from build123d import *

# Parameters (mm, degrees)
SKETCH1_W             = 8
SKETCH1_H             = 36
SKETCH1_R             = 1.25
BOSS_EXTRUDE1_DEPTH   = 5
BOSS_EXTRUDE1_2_DEPTH = 5
SKETCH2_W             = 54
SKETCH2_H             = 5
BOSS_EXTRUDE2_DEPTH   = 12
SKETCH4_W             = 54
SKETCH4_H             = 12
BOSS_EXTRUDE3_DEPTH   = 64
SKETCH5_W             = 40.6
SKETCH5_H             = 60.5
CUT_EXTRUDE1_DEPTH    = 10
BOSS_EXTRUDE4_DEPTH   = 3
BOSS_EXTRUDE5_START   = -54
BOSS_EXTRUDE5_DEPTH   = 3
CHAMFER1_SIZE         = 2
CHAMFER2_SIZE         = 1
CHAMFER3_SIZE         = 3
SKETCH8_W             = 66
SKETCH8_H             = 71
BOSS_EXTRUDE6_DEPTH   = 3
SKETCH9_W             = 3
SKETCH9_H             = 46
SKETCH9_W_2           = 4
SKETCH9_H_2           = 71
BOSS_EXTRUDE7_DEPTH   = 6
BOSS_EXTRUDE8_DEPTH   = 40
SKETCH12_W            = 2.5
SKETCH12_H            = 71
BOSS_EXTRUDE9_DEPTH   = 3
CHAMFER4_SIZE         = 5


with BuildPart() as part:
    # Sketch1 → Boss-Extrude1 (new body)
    with BuildSketch(Plane.XY):
        with Locations((1, 15)):
            Rectangle(SKETCH1_W, SKETCH1_H)
        Circle(SKETCH1_R, mode=Mode.SUBTRACT)
        with Locations((0, 30)):
            Circle(SKETCH1_R, mode=Mode.SUBTRACT)
    extrude(amount=BOSS_EXTRUDE1_DEPTH)



with BuildPart() as body_2:
    # Sketch1 → Boss-Extrude1 2 (new body)
    with BuildSketch(Plane.XY):
        with Locations((47, 15)):
            Rectangle(SKETCH1_W, SKETCH1_H)
        with Locations((48, 0)):
            Circle(SKETCH1_R, mode=Mode.SUBTRACT)
        with Locations((48, 30)):
            Circle(SKETCH1_R, mode=Mode.SUBTRACT)
    extrude(amount=BOSS_EXTRUDE1_2_DEPTH)


with BuildPart() as part_1:
    add(part.part)

    add(body_2.part)  # Boss-Extrude2 merges body 2
    # Sketch2 → Boss-Extrude2 (add)
    with BuildSketch(Plane.XZ.offset(3)):
        with Locations((24, 2.5)):
            Rectangle(SKETCH2_W, SKETCH2_H)
    extrude(amount=BOSS_EXTRUDE2_DEPTH)

    # Sketch4 → Boss-Extrude3 (add)
    with BuildSketch(Plane.XY.offset(5)):
        with Locations((24, -9)):
            Rectangle(SKETCH4_W, SKETCH4_H)
    extrude(amount=BOSS_EXTRUDE3_DEPTH)

    # Sketch5 → Cut-Extrude1 (cut)
    with BuildSketch(Plane(origin=(0, -3, 0), x_dir=(1, 0, 0), z_dir=(0, 1, 0))):
        with Locations((24, -39.25)):
            Rectangle(SKETCH5_W, SKETCH5_H)
    extrude(amount=-CUT_EXTRUDE1_DEPTH, mode=Mode.SUBTRACT)

    # Sketch7 → Boss-Extrude4 (add)
    with BuildSketch(Plane.ZY.offset(3)):
        Polygon((0, 33), (0, -15), (48, -15), (48, -3), (5, 33), align=None)
    extrude(amount=BOSS_EXTRUDE4_DEPTH)

    # Sketch7<2> → Boss-Extrude5 (add)
    with BuildSketch(Plane.ZY.offset(3).offset(BOSS_EXTRUDE5_START)):
        Polygon((0, 33), (0, -15), (48, -15), (48, -3), (5, 33), align=None)
    extrude(amount=-BOSS_EXTRUDE5_DEPTH)

    # Chamfer1
    chamfer1_edges = [part_1.edges().sort_by_distance(p)[0] for p in [
        (-3, -9, 69),
        (51, -9, 69),
        (-6, 9, 0),
        (54, 9, 0),
    ]]
    chamfer(chamfer1_edges, length=CHAMFER1_SIZE)

    # Chamfer2
    chamfer2_edges = [part_1.edges().sort_by_distance(p)[0] for p in [
        (44.3, -3, 39),
        (24, -3, 9),
        (3.7, -3, 39),
    ]]
    chamfer(chamfer2_edges, length=CHAMFER2_SIZE)

    # Chamfer3
    # the kernel refuses this chamfer: 3 mm, written as the material it adds along each edge
    with BuildSketch(Plane(origin=(51, -15, 48), x_dir=(-0.027495876610584467, 0, 0.9996219169112969), z_dir=(0, 1, 0))) as chamfer3_piece_1_section:
        Polygon((CHAMFER3_SIZE * 0.999621916911, CHAMFER3_SIZE * 0.0274958766106), (-CHAMFER3_SIZE * 0.0274958766106, CHAMFER3_SIZE * 0.999621916911), (0, 0), align=None)
    chamfer3_piece_1 = extrude(amount=12, mode=Mode.PRIVATE)
    chamfer3_piece_1 = split(chamfer3_piece_1, bisect_by=Plane(origin=(54, -9.397887016, 48.948587344), z_dir=(-1, 0, 0)), keep=Keep.TOP, mode=Mode.PRIVATE)
    chamfer3_piece_1 = split(chamfer3_piece_1, bisect_by=Plane(origin=(52.008422093, -6.10336241, 51.70679399), z_dir=(0, -0.7667576729931039, -0.6419366564593428)), keep=Keep.TOP, mode=Mode.PRIVATE)
    add(chamfer3_piece_1)
    with BuildSketch(Plane(origin=(51, -15, 48), x_dir=(-0.027495876610584467, 0, 0.9996219169112969), z_dir=(0, 1, 0))) as chamfer3_piece_2_section:
        Polygon((CHAMFER3_SIZE * 0.999621916911, CHAMFER3_SIZE * 0.0274958766106), (-CHAMFER3_SIZE * 0.0274958766106, CHAMFER3_SIZE * 0.999621916911), (0, 0), align=None)
    chamfer3_piece_2 = extrude(amount=12, mode=Mode.PRIVATE)
    chamfer3_piece_2 = split(chamfer3_piece_2, bisect_by=Plane(origin=(51.683373084, -4.039508932, 49.241635668), z_dir=(0, 0.7667576729931039, 0.6419366564593428)), keep=Keep.TOP, mode=Mode.PRIVATE)
    add(chamfer3_piece_2)
    with BuildSketch(Plane(origin=(-3, -15, 48), x_dir=(0.027495876610586334, 0, 0.9996219169112968), z_dir=(0, 1, 0))) as chamfer3_piece_3_section:
        Polygon((CHAMFER3_SIZE * 0.999621916911, -CHAMFER3_SIZE * 0.0274958766106), (-CHAMFER3_SIZE * 0.0274958766106, -CHAMFER3_SIZE * 0.999621916911), (0, 0), align=None)
    chamfer3_piece_3 = extrude(amount=12, mode=Mode.PRIVATE)
    chamfer3_piece_3 = split(chamfer3_piece_3, bisect_by=Plane(origin=(-6, -9.397887016, 48.948587344), z_dir=(1, 0, 0)), keep=Keep.TOP, mode=Mode.PRIVATE)
    chamfer3_piece_3 = split(chamfer3_piece_3, bisect_by=Plane(origin=(-4.008422093, -6.10336241, 51.70679399), z_dir=(0, -0.7667576729931039, -0.6419366564593428)), keep=Keep.TOP, mode=Mode.PRIVATE)
    add(chamfer3_piece_3)
    with BuildSketch(Plane(origin=(-3, -15, 48), x_dir=(0.027495876610586334, 0, 0.9996219169112968), z_dir=(0, 1, 0))) as chamfer3_piece_4_section:
        Polygon((CHAMFER3_SIZE * 0.999621916911, -CHAMFER3_SIZE * 0.0274958766106), (-CHAMFER3_SIZE * 0.0274958766106, -CHAMFER3_SIZE * 0.999621916911), (0, 0), align=None)
    chamfer3_piece_4 = extrude(amount=12, mode=Mode.PRIVATE)
    chamfer3_piece_4 = split(chamfer3_piece_4, bisect_by=Plane(origin=(-3.683373084, -4.039508932, 49.241635668), z_dir=(0, 0.7667576729931039, 0.6419366564593428)), keep=Keep.TOP, mode=Mode.PRIVATE)
    add(chamfer3_piece_4)
    with BuildSketch(Plane(origin=(-3, 33, 5), x_dir=(-0.02749587661058635, 0, 0.9996219169112968), z_dir=(0, -1, 0))) as chamfer3_piece_5_section:
        Polygon((CHAMFER3_SIZE * 0.999621916911, -CHAMFER3_SIZE * 0.0274958766106), (-CHAMFER3_SIZE * 0.0274958766106, -CHAMFER3_SIZE * 0.999621916911), (0, 0), align=None)
    chamfer3_piece_5 = extrude(amount=43.715048964, mode=Mode.PRIVATE)
    chamfer3_piece_5 = split(chamfer3_piece_5, bisect_by=Plane(origin=(-2.02772284, 24.92424675, 14.646038604), z_dir=(0, -0.7667576729931039, -0.6419366564593428)), keep=Keep.TOP, mode=Mode.PRIVATE)
    chamfer3_piece_5 = chamfer3_piece_5 - Plane(origin=(0, 0, 5.988374144), x_dir=(1, 0, 0), z_dir=(0, 0, -1)) * Cylinder(1.25, 100, mode=Mode.PRIVATE)
    chamfer3_piece_5 = chamfer3_piece_5 - Plane(origin=(0, 30, 5.988374144), x_dir=(1, 0, 0), z_dir=(0, 0, -1)) * Cylinder(1.25, 100, mode=Mode.PRIVATE)
    add(chamfer3_piece_5)
    with BuildSketch(Plane(origin=(51, -10.715048964, 5), x_dir=(0.02749587661058678, 0, 0.9996219169112968), z_dir=(0, 1, 0))) as chamfer3_piece_6_section:
        Polygon((CHAMFER3_SIZE * 0.999621916911, -CHAMFER3_SIZE * 0.0274958766106), (-CHAMFER3_SIZE * 0.0274958766106, -CHAMFER3_SIZE * 0.999621916911), (0, 0), align=None)
    chamfer3_piece_6 = extrude(amount=43.715048964, mode=Mode.PRIVATE)
    chamfer3_piece_6 = split(chamfer3_piece_6, bisect_by=Plane(origin=(50.01061912, 16.088421834, 25.199940587), z_dir=(0, -0.7667576729931039, -0.6419366564593428)), keep=Keep.TOP, mode=Mode.PRIVATE)
    chamfer3_piece_6 = chamfer3_piece_6 - Plane(origin=(48, 0, 5.98938088), x_dir=(1, 0, 0), z_dir=(0, 0, -1)) * Cylinder(1.25, 100, mode=Mode.PRIVATE)
    chamfer3_piece_6 = chamfer3_piece_6 - Plane(origin=(48, 30, 5.98938088), x_dir=(1, 0, 0), z_dir=(0, 0, -1)) * Cylinder(1.25, 100, mode=Mode.PRIVATE)
    add(chamfer3_piece_6)

    # Sketch8 → Boss-Extrude6 (add)
    with BuildSketch(Plane.XZ.offset(15)):
        with Locations((82, 35.5)):
            Rectangle(SKETCH8_W, SKETCH8_H)
    extrude(amount=-BOSS_EXTRUDE6_DEPTH)

    # Sketch9 → Boss-Extrude7 (add)
    with BuildSketch(Plane(origin=(0, -12, 0), x_dir=(1, 0, 0), z_dir=(0, 1, 0))):
        with Locations((55.5, -25)):
            Rectangle(SKETCH9_W, SKETCH9_H)
        with Locations((113, -35.5)):
            Rectangle(SKETCH9_W_2, SKETCH9_H_2)
    extrude(amount=BOSS_EXTRUDE7_DEPTH)

    # Sketch11 → Boss-Extrude8 (add)
    with BuildSketch(Plane(origin=(0, 0, 2), x_dir=(-1, 0, 0), z_dir=(0, 0, -1))):
        with BuildLine():
            Line((-54, -1.45), (-54, -4.65))
            ThreePointArc((-54, -4.65), (-54.8, -3.05), (-54, -1.45))
        make_face()
    extrude(amount=-BOSS_EXTRUDE8_DEPTH)

    # Sketch12 → Boss-Extrude9 (add)
    with BuildSketch(Plane(origin=(0, -6, 0), x_dir=(1, 0, 0), z_dir=(0, 1, 0))):
        with Locations((113.75, -35.5)):
            Rectangle(SKETCH12_W, SKETCH12_H)
    extrude(amount=BOSS_EXTRUDE9_DEPTH)

    # Chamfer4
    # the kernel refuses this chamfer: 5 mm, written as the material it takes off along each edge
    with BuildSketch(Plane(origin=(115, -12, 0), x_dir=(-0.9996219169112968, 0, -0.027495876610586334), z_dir=(0, 1, 0))) as chamfer4_piece_1:
        Polygon((CHAMFER4_SIZE * 0.999621916911, CHAMFER4_SIZE * 0.0274958766106), (-CHAMFER4_SIZE * 0.0274958766106, CHAMFER4_SIZE * 0.999621916911), (0, 0), align=None)
    extrude(amount=6, mode=Mode.SUBTRACT)
    with BuildSketch(Plane(origin=(115, -12, 71), x_dir=(-0.9996219169112968, 0, 0.027495876610587663), z_dir=(0, 1, 0))) as chamfer4_piece_2:
        Polygon((CHAMFER4_SIZE * 0.999621916911, -CHAMFER4_SIZE * 0.0274958766106), (-CHAMFER4_SIZE * 0.0274958766106, -CHAMFER4_SIZE * 0.999621916911), (0, 0), align=None)
    extrude(amount=6, mode=Mode.SUBTRACT)
    with BuildSketch(Plane(origin=(115, -27.85841494, 71), x_dir=(-0.9996219169112968, 0, 0.027495876610587663), z_dir=(0, 1, 0)), Plane(origin=(115, -6, 71), x_dir=(-0.9996219169112968, 0, 0.027495876610587663), z_dir=(0, 1, 0))) as chamfer4_piece_3:
        Polygon((CHAMFER4_SIZE * 0.999621916911, -CHAMFER4_SIZE * 0.0274958766106), (-CHAMFER4_SIZE * 0.0274958766106, -CHAMFER4_SIZE * 0.999621916911), (0, 0), align=None)
    extrude(amount=15.85841494, mode=Mode.SUBTRACT)
    with BuildSketch(Plane(origin=(115, -27.85841494, 0), x_dir=(-0.9996219169112968, 0, -0.02749587661058646), z_dir=(0, 1, 0)), Plane(origin=(115, -6, 0), x_dir=(-0.9996219169112968, 0, -0.02749587661058634), z_dir=(0, 1, 0))) as chamfer4_piece_4:
        Polygon((CHAMFER4_SIZE * 0.999621916911, CHAMFER4_SIZE * 0.0274958766106), (-CHAMFER4_SIZE * 0.0274958766106, CHAMFER4_SIZE * 0.999621916911), (0, 0), align=None)
    extrude(amount=15.85841494, mode=Mode.SUBTRACT)


solid = part_1.part
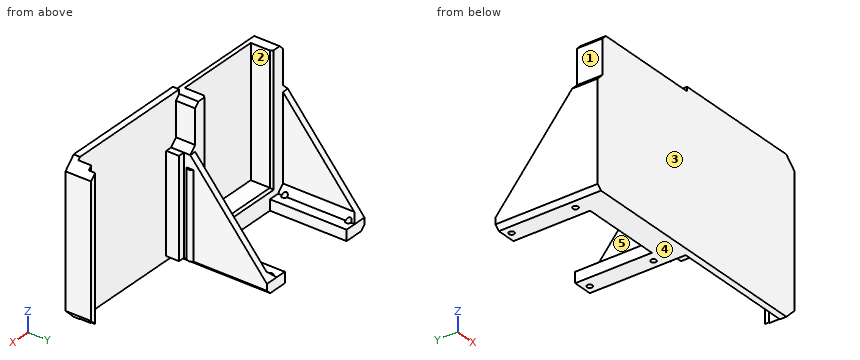
Geometry: final body of the model. Coordinates: model frame, mm. Face numbers are marked on the shaded views. A direction names the side the tool comes from. Round coordinates to 2 decimals unless told otherwise and drop trailing zeros. Order: outer loops, then holes, each group sorted by start corner. A loop starts at its lowest first (then second) coordinate and runs counter-clockwise, first axis right, second up. Notation, with made-up numbers: (-32, 54) -> (5, 54) arc R13 cw to (5, 59) -> close; hole circle Ø8 at (16.5, 60.5). An arc over 180 degrees is marked (long way). Put each result on its own line as item: value. Start each with the question number.
Q1. First-contact query: pin 1 (4 mm diameter, centred on x = 3.5, y = 17, fed in from +Z); pin 2 (1.5 mm diameter, centred on x = 0, y = 30, fed in from -Z); pin 3 (3.5 mm diameter, centred on x = 16, y = -12, fed in from +Z); pin 4 (1 mm diameter, centred on y = -13.5, z = 70, fed in from -X). Flat tips, straight axial feed; report the tip coordinate or a pass-through.
Q2. Line query: probe 1 along X at (y, z) = (30, 3.45); probe 2 along X at (y, z) = (-11, 38); probe 3 along Y at (x, z) = (48, 1.75). Output: solid intervals per line, ascending.
Q3. Section A-A on y = 15. Return the cut outline in (x, z), and give its area (3 significant figures).
Q4. Section C-C on z = 23. Return the cut outline in (x, y).
Q5. Reachability of the marked faces 4 and 5 from +Z, -Z, +X, -X, +Y, -Y: full face, straight path, thin tool, end or side. Return the list, or none.
Q6. Section D-D on y = 7.5. Return the cut outline in (x, z), and give its area (3 significant figures).
Q7. Section B-B on y = 0. Return the cut outline in (x, z), and give its area (3 significant figures).
Q8. Pull-direction query (X, two-part tool) for the marked faces 1, 2 and 3; classes: +X half, -X half, draft (parallel to the pull), parting line (faces both ways), or undercut.
Ans:
1. pin 1: stops at z = 5
1. pin 2: passes through
1. pin 3: stops at z = 69
1. pin 4: stops at x = 49
2. probe 1: x = -6 to -1.25, 1.25 to 5, 43 to 46.75, 49.25 to 54
2. probe 2: x = -6 to 3.7, 44.3 to 57, 111 to 115
2. probe 3: y = -15 to -1.25, 1.25 to 28.75, 31.25 to 33
3. outline: (-6, 2) -> (-4, 0) -> (5, 0) -> (5, 5) -> (0, 5) -> (-3, 8) -> (-3, 26.5) -> (-6, 26.5) -> close; (43, 0) -> (52, 0) -> (54, 2) -> (54, 26.5) -> (51, 26.5) -> (51, 8) -> (48, 5) -> (43, 5) -> close
3. area: 244 mm2
4. outline: (-6, -15) -> (115, -15) -> (115, -3) -> (112.5, -3) -> (112.5, -6) -> (111, -6) -> (111, -12) -> (57, -12) -> (57, -6) -> (54, -6) -> (54, -4.65) arc R2 ccw to (54, -1.45) -> (54, 17.93) -> (51, 17.93) -> (51, -3) -> (45.3, -3) -> (44.3, -4) -> (44.3, -13) -> (3.7, -13) -> (3.7, -4) -> (2.7, -3) -> (-3, -3) -> (-3, 17.93) -> (-6, 17.93) -> close
5. face 4: -Z, +X, -X, +Y, -Y
5. face 5: +Z, +Y
6. outline: (-6, 2) -> (-4, 0) -> (5, 0) -> (5, 5) -> (0, 5) -> (-3, 8) -> (-3, 35.46) -> (-6, 35.46) -> close; (43, 0) -> (52, 0) -> (54, 2) -> (54, 35.46) -> (51, 35.46) -> (51, 8) -> (48, 5) -> (43, 5) -> close
6. area: 298 mm2
7. outline: (-6, 2) -> (-4, 0) -> (-1.25, 0) -> (-1.25, 6.25) -> (-3, 8) -> (-3, 44.42) -> (-6, 44.42) -> close; (1.25, 0) -> (5, 0) -> (5, 5) -> (1.25, 5) -> close; (43, 0) -> (46.75, 0) -> (46.75, 5) -> (43, 5) -> close; (49.25, 0) -> (52, 0) -> (54, 2) -> (54, 44.42) -> (51, 44.42) -> (51, 8) -> (49.25, 6.25) -> close
7. area: 325 mm2
8. face 1: -X half
8. face 2: undercut
8. face 3: draft
